```python
from build123d import *

# Parameters (mm, degrees)
F1_DEPTH = 100


with BuildPart() as f1:
    # F0 (on Right) → F1 (new body)
    with BuildSketch(Plane.YZ):
        Polygon((200, 136.370988), (0, 10), (15.826417, 10), (200, 126.370988), align=None)
        Polygon((0, 10), (0, 0), (15.826417, 10), align=None)
        Polygon((15.826417, 10), (0, 0), (200, 0), (200, 10), align=None)
    extrude(amount=F1_DEPTH)


solid = f1.part
```
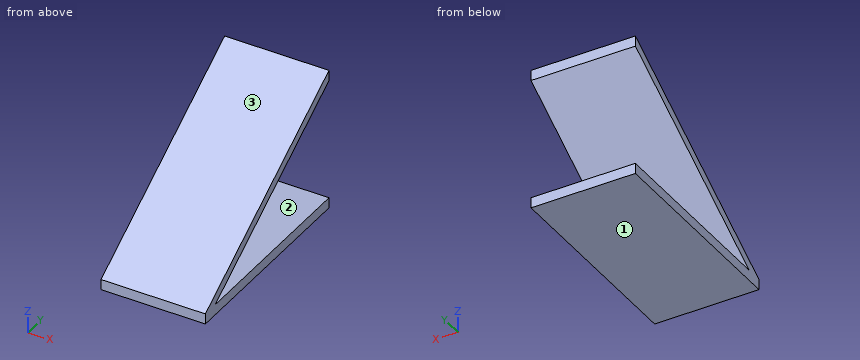
Geometry check sheet. Reference: the model listing, model coordinates, mm. Face numbers are marked on the shaded views. Coordinates: 2 decimals unless noted, no trailing zeros. Loops run counter-clockwise (first coordinate to the right, second up) from the corner with the lowest first, then second, coordinate; pieces in that order, holes last.
Item 1: Thickness scan on line 1 (Z direction, x = 84.5, y = 115); line 2 (Z direction, x = 39.5, y = 98); line 3 (Y direction, x = 55, z = 60.5). Record the ranges inside material, lowest first.
Item 2: Release check for a two-part mould opening along Z. For the marked faces 1, 2 and 3 record: released by +Z, released by -Z, zero draft, split by the parting line, or undercut.
Item 3: Sectioned sample at B-B, the plane y = 157. Record the boundary of the cut face in (x, z), then the cut area to 3 significant figures.
Item 4: Go/stop test with flat-tipped pins: pin 1 Ø1 at (x, z) = (88.5, 41.5) entering from -Y; pin 2 Ø12 at (x, z) = (61, 30.5) entering from +Y; pin 3 Ø2 at (x, y) = (73, 78.5) entering from +Z. Record where each tip stops, or that it passes through.
Item 5: Sectioned sample at A-A, the plane x = 79.5. Record the boundary of the cut face in (y, z), then the cut area to 3 significant figures.
Item 6: Sectioned sample at C-C, the plane z = 79.5. Record the boundary of the cut face in (x, y).
Check result:
1. line 1: z = 0 to 10, 72.66 to 82.66
1. line 2: z = 0 to 10, 61.92 to 71.92
1. line 3: y = 79.92 to 95.75
2. face 1: released by -Z
2. face 2: undercut
2. face 3: released by +Z
3. outline: (0, 0) - (100, 0) - (100, 10) - (0, 10) - close; (0, 99.2) - (100, 99.2) - (100, 109.2) - (0, 109.2) - close
3. area: 2,000 mm2
4. pin 1: stops at y = 49.06
4. pin 2: stops at y = 57.77
4. pin 3: stops at z = 60.23
5. outline: (0, 0) - (200, 0) - (200, 10) - (15.83, 10) - (200, 126.37) - (200, 136.37) - (0, 10) - close
5. area: 3,920 mm2
6. outline: (0, 109.99) - (100, 109.99) - (100, 125.82) - (0, 125.82) - close
